Source: CAD feature listing. Evaluate the final solid. Frame: model axes, mm. A direction names the side the tool comes from. Coordinates: 2 decimals unless noted, no trailing zeros. Write each loop counter-clockwise with the first axis right and the second up, starting at its lowest first coordinate (ties: lowest second). Pieces come first, ordered by that corner, then holes. Notation, with made-up numbers: (49, 14.5) - (89, 14.5) arc R13 cw to (89, 33.5) - close; hole circle Ø7 at (-21, 86). An arc over 180 degrees is marked (long way). One line per item, written item: value.
from build123d import *

# Parameters (mm, degrees)
ESQUISSE1_W                = 53
ESQUISSE1_H                = 50
BOSS_EXTRU_1_DEPTH         = 3
ESQUISSE2_W                = 3
ESQUISSE2_H                = 50
BOSS_EXTRU_2_DEPTH         = 48
ESQUISSE3_R                = 11.05
ESQUISSE3_R_2              = 1.75
ENL_V_MAT_EXTRU_1_DEPTH    = 49
CHANFREIN1_SIZE            = 5
BOSS_EXTRU_3_DEPTH         = 3
R_P_TITION_LIN_AIRE1_COUNT = 2
R_P_TITION_LIN_AIRE1_PITCH = 47
CONG_3_R                   = 1.5


with BuildPart() as part:
    # Esquisse1 → Boss.-Extru.1 (new body)
    with BuildSketch(Plane.XY):
        with Locations((53.536991909, -25)):
            Rectangle(ESQUISSE1_W, ESQUISSE1_H)
        with BuildLine():
            Line((39.036991909, -10.508361759), (69.036991909, -10.508361759))
            ThreePointArc((69.036991909, -10.508361759), (71.136991909, -8.408361759), (69.036991909, -6.308361759))
            Line((69.036991909, -6.308361759), (39.036991909, -6.308361759))
            ThreePointArc((39.036991909, -6.308361759), (36.936991909, -8.408361759), (39.036991909, -10.508361759))
        make_face(mode=Mode.SUBTRACT)
        with BuildLine():
            Line((39.036991909, -36.308361759), (69.036991909, -36.308361759))
            ThreePointArc((69.036991909, -36.308361759), (71.136991909, -38.408361759), (69.036991909, -40.508361759))
            Line((69.036991909, -40.508361759), (39.036991909, -40.508361759))
            ThreePointArc((39.036991909, -40.508361759), (36.936991909, -38.408361759), (39.036991909, -36.308361759))
        make_face(mode=Mode.SUBTRACT)
    extrude(amount=BOSS_EXTRU_1_DEPTH)

    # Esquisse2 → Boss.-Extru.2 (add)
    with BuildSketch(Plane.XY.offset(3)):
        with Locations((28.536991909, -25)):
            Rectangle(ESQUISSE2_W, ESQUISSE2_H)
    extrude(amount=BOSS_EXTRU_2_DEPTH)

    # Esquisse3 → Enlèv. mat.-Extru.1 (cut)
    with BuildSketch(Plane.ZY.offset(-27.036991909)):
        with Locations(Location((30, -25, 0), (0, 0, 270))):
            Circle(ESQUISSE3_R)
        with Locations(Location((14.5, -9.5, 0), (0, 0, 270))):
            Circle(ESQUISSE3_R_2)
        with Locations(Location((45.5, -9.5, 0), (0, 0, 270))):
            Circle(ESQUISSE3_R_2)
        with Locations(Location((45.5, -40.5, 0), (0, 0, 270))):
            Circle(ESQUISSE3_R_2)
        with Locations(Location((14.5, -40.5, 0), (0, 0, 270))):
            Circle(ESQUISSE3_R_2)
    extrude(amount=-ENL_V_MAT_EXTRU_1_DEPTH, mode=Mode.SUBTRACT)

    # Chanfrein1
    chanfrein1_edges = [part.edges().sort_by_distance(p)[0] for p in [
        (80.036991909, -50, 1.5),
        (80.036991909, 0, 1.5),
        (28.536991909, -50, 51),
        (28.536991909, 0, 51),
    ]]
    chamfer(chanfrein1_edges, length=CHANFREIN1_SIZE)

    # Esquisse4 → Boss.-Extru.3 (add)
    with BuildSketch(Plane.XZ.offset(50)):
        Polygon((30.036991909, 5), (32.036991909, 3), (43.036991909, 3), (30.036991909, 23), align=None)
    boss_extru_3 = extrude(amount=-BOSS_EXTRU_3_DEPTH)

    # Répétition linéaire1: Boss.-Extru.3 ×2
    with Locations(*[(0, i * R_P_TITION_LIN_AIRE1_PITCH, 0) for i in range(1, R_P_TITION_LIN_AIRE1_COUNT)]):
        add(boss_extru_3)

    # Congé3
    cong_3_edges = [part.edges().sort_by_distance(p)[0] for p in [
        (27.036991909, -25, 0),
        (30.036991909, -25, 3),
    ]]
    fillet(cong_3_edges, radius=CONG_3_R)


solid = part.part
1) Section query C-C on z = 30. Output: boundary loops of the cut face in (x, y).
Values found:
outline: (27.04, -50) - (30.04, -50) - (30.04, -36.05) - (27.04, -36.05) - close; (27.04, -13.95) - (30.04, -13.95) - (30.04, 0) - (27.04, 0) - close
2) Contact query for flat-ended pins moving along their axis: P1, Ø14.5, axis at x = 48, y = -33.5, coming from the +Z side; P2, Ø23, axis at y = -24, z = 32, coming from the +X side; P3, Ø3, axis at y = -9.5, z = 45.5, coming from the -X side. Output: stop coordinate, or through.
Values found:
P1: z = 3
P2: x = 30.04
P3: through
3) Material intervals for line 1 (Y direction, x = 28, z = 45); line 2 (Z direction, x = 28, y = -9); line 3 (Z direction, x = 29, y = -9), sorted ascending.
Values found:
line 1: -50 to -42.18, -38.82 to -11.18, -7.82 to 0
line 2: 0.1 to 12.82, 16.18 to 43.82, 47.18 to 51
line 3: 0 to 12.82, 16.18 to 43.82, 47.18 to 51
4) Reachability of faces 1 (the flat face through (34, -3, 9)), 2 (the flat face through (54, -40.508, 1)), 3 (the cylindrical face through (27.465, -24.65, 0.451)) from +Z, -Z, +X, -X, +Y, -Y: full face, straight path, thin tool, end or side. Return the list, or none.
Values found:
face 1: +Z, +X
face 2: +Z, -Z
face 3: -Z, -X, +Y, -Y
5) Section query B-B on y = -25. Output: boundary loops of the cut face in (x, z), then the cut area to 3 significant figures.
Values found:
outline: (27.04, 1.5) arc R1.5 ccw to (28.54, 0) - (80.04, 0) - (80.04, 3) - (31.54, 3) arc R1.5 cw to (30.04, 4.5) - (30.04, 18.95) - (27.04, 18.95) - close; (27.04, 41.05) - (30.04, 41.05) - (30.04, 51) - (27.04, 51) - close
area: 237 mm2
6) Section query D-D on y = -9.5. Output: boundary loops of the cut face in (x, z).
Values found:
outline: (27.04, 1.5) arc R1.5 ccw to (28.54, 0) - (37.24, 0) - (37.24, 3) - (31.54, 3) arc R1.5 cw to (30.04, 4.5) - (30.04, 12.75) - (27.04, 12.75) - close; (27.04, 16.25) - (30.04, 16.25) - (30.04, 43.75) - (27.04, 43.75) - close; (27.04, 47.25) - (30.04, 47.25) - (30.04, 51) - (27.04, 51) - close; (70.83, 0) - (80.04, 0) - (80.04, 3) - (70.83, 3) - close
7) Draft query along Y for faces 4 (the flat face through (36.6, -1.5, 12.9)), 5 (the flat face through (55, -25, 3)), 6 (the flat face through (77.572, -47.465, 1.479)), 7 (the cylindrical face through (28.5, -10.4, 16)). Return one class per face: released by +Y, released by -Y, zero draft, split by the parting line, or undercut.
Values found:
face 4: zero draft
face 5: undercut
face 6: released by -Y
face 7: undercut
8) Section query A-A on x = 48. Output: boundary loops of the cut face in (y, z).
Values found:
outline: (-50, 0) - (-40.51, 0) - (-40.51, 3) - (-50, 3) - close; (-36.31, 0) - (-10.51, 0) - (-10.51, 3) - (-36.31, 3) - close; (-6.31, 0) - (0, 0) - (0, 3) - (-6.31, 3) - close
